Read the model definition and answer for the solid it produces. Units are mm, in the model's axes. A direction names the side the tool comes from. Round coordinates to 2 decimals unless told otherwise and drop trailing zeros. Loops run counter-clockwise (first coordinate to the right, second up) from the corner with the lowest first, then second, coordinate; pieces in that order, holes last. Notation, with made-up numbers: M -3,24.25 L 14,24.25 A17 ccw 14,49.25 Z; hole C 65.5,-6 d8. An arc over 180 degrees is marked long. Write each question's results on one line, items separated by ' | '.
from build123d import *

# Parameters (mm, degrees)
SKETCH1_W           = 160
SKETCH1_H           = 150
BOSS_EXTRUDE1_DEPTH = 15
BOSS_EXTRUDE2_DEPTH = 5
CUT_EXTRUDE1_DEPTH  = 5


with BuildPart() as part:
    # Sketch1 → Boss-Extrude1 (new body)
    with BuildSketch(Plane.XY):
        with Locations((0, 8.754863813)):
            Rectangle(SKETCH1_W, SKETCH1_H)
    extrude(amount=BOSS_EXTRUDE1_DEPTH)

    # Sketch2 → Boss-Extrude2 (add)
    with BuildSketch(Plane(origin=(80, 0, 0), x_dir=(0, 0, -1), z_dir=(1, 0, 0))):
        with BuildLine():
            Line((-10, -58.745136187), (-10, 89.520228405))
            ThreePointArc((-10, 89.520228405), (-7.5, 92.020228405), (-5, 89.520228405))
            Line((-5, 89.520228405), (-5, -58.745136187))
            ThreePointArc((-5, -58.745136187), (-7.5, -61.245136187), (-10, -58.745136187))
        make_face()
    boss_extrude2 = extrude(amount=BOSS_EXTRUDE2_DEPTH)

    # Mirror1: Boss-Extrude2 across plane
    add(boss_extrude2.mirror(Plane(origin=(0, 0, 0), x_dir=(0, 0, 1), z_dir=(1, 0, 0))))

    # Sketch3 → Cut-Extrude1 (cut)
    with BuildSketch(Plane.ZY.offset(85)):
        with BuildLine():
            Line((5, 83.754863813), (10, 83.754863813))
            Line((10, 83.754863813), (10, 89.520228405))
            ThreePointArc((10, 89.520228405), (7.5, 92.020228405), (5, 89.520228405))
            Line((5, 89.520228405), (5, 83.754863813))
        make_face()
    cut_extrude1 = extrude(amount=-CUT_EXTRUDE1_DEPTH, mode=Mode.SUBTRACT)

    # Mirror2: Cut-Extrude1 across plane
    add(cut_extrude1.mirror(Plane(origin=(0, 0, 0), x_dir=(0, 0, 1), z_dir=(1, 0, 0))), mode=Mode.SUBTRACT)


solid = part.part
Item 1: The part is cut by section B-B (z = 13). Determine the outline of the cut face in (x, y), plus the area to 3 significant figures.
Outcome:
outline: M -80,-66.25 L 80,-66.25 L 80,83.75 L -80,83.75 Z | area: 24,000 mm2
Item 2: A straight line is drawn through the part: line 1 (X direction, y = -13, z = 1). Find the intervals that lie inside material, in ascending order.
Outcome:
line 1: x = -80 to 80
Item 3: The part is cut by section A-A (y = 25). Determine the outline of the cut face in (x, z), plus the area to 3 significant figures.
Outcome:
outline: M -85,5 L -80,5 L -80,0 L 80,0 L 80,5 L 85,5 L 85,10 L 80,10 L 80,15 L -80,15 L -80,10 L -85,10 Z | area: 2,450 mm2
Item 4: Flat-ended cylindrical pins translate along their axes: pin 1 (1.5 mm diameter, centred on x = 81.5, y = 29.5, fed in from -Z); pin 2 (1.5 mm diameter, centred on x = 83, y = 34, fed in from +Z). Find the tip coordinate at first contact, or state that the pin passes through.
Outcome:
pin 1: stops at z = 5 | pin 2: stops at z = 10
Item 5: For faces 1 (the face through (-82, 12, 10)), 2 (the face through (82, 14, 5)), 3 (the face through (-82.465, -61.245, 7.445)), determine the directions among +Z, -Z, +X, -X, +Y, -Y from which every point of the face is accessible in a straight line to the end or side of a thin tool.
Outcome:
face 1: +Z, -X, +Y, -Y | face 2: -Z, +X, +Y, -Y | face 3: -X, -Y
